Design review of the part built by this model. Coordinates are the model's own, in mm. Face numbers are marked on the shaded views. A direction names the side the tool comes from. Give positions to 0.01 mm unless a question says otherwise; leave off trailing zeros. Loops run counter-clockwise (first coordinate to the right, second up) from the corner with the lowest first, then second, coordinate; pieces in that order, holes last. Notation, with made-up numbers: M -35.5,10.5 L -0.5,10.5 A14 cw -0.5,18.5 Z; hole C 69.5,69.5 d3. An arc over 180 degrees is marked long. Use a Markdown table: item, result. Add a question column.
(1) For probe 1 along X at (y, z) = (11.5, 156.5); probe 2 along Y at (x, z) = (39, -132); probe 3 along Y at (x, z) = (3.5, -138), list the stretches that pass through material, from the lowest coordinate up.
(2) Insertion check: pin 1 Ø1.5 at (x, y) = (26.5, 24.5) entering from -Z; pin 2 Ø1 at (x, y) = (15.5, 28.5) entering from -Z; pin 3 Ø4 at (x, y) = (28.5, -8) entering from +Z. Each pin has a flat end and moves straight along its axis. Give the tip position at first contact, or say it passes through.
(3) For the marked faces 4 and 5, list the 3-axis set-ups (+Z, -Z, +X, -X, +Y, -Y) from which the entire face can be reached by the end or side of a thin tool; tool diameter is ignored.
(4) Add section C-C, the plane y = 27.5. Give the boundary of the cut face in (x, z), then the cut area to 3 significant figures.
(5) Draft analysis for pull direction X (two halves, no side actions). For the marked faces 1, 2 and 3, state which applies: pulls with the +X half, pulls with the -X half, needs draft (parallel to the pull), parting line crosses it, or undercut.
(6) Add section B-B, the plane x = 45.5. Give the boundary of the cut face in (y, z).
(7) Add section D-D, the plane x = 16. Give the boundary of the cut face in (y, z), then the cut area to 3 significant figures.
(8) Add section A-A, the plane z = 120.5. Give the boundary of the cut face in (x, y), then the cut area to 3 significant figures.
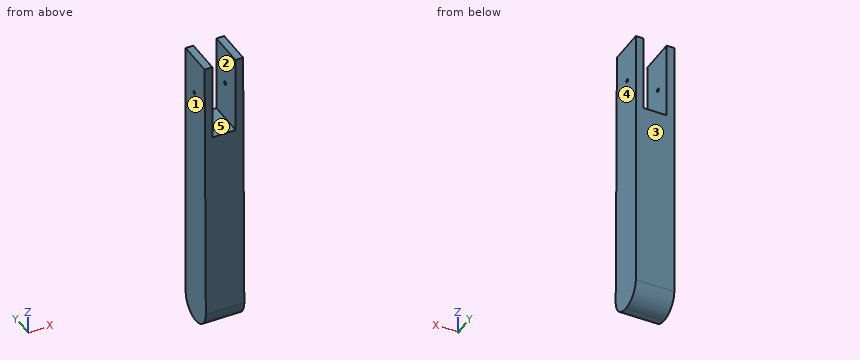
```python
from build123d import *

# Parameters (mm, degrees)
BOSS_EXTRUDE1_DEPTH = 50
SKETCH6_W           = 30
SKETCH6_H           = 100
CUT_EXTRUDE3_DEPTH  = 222.479310794
SKETCH5_R           = 2.25
CUT_EXTRUDE2_DEPTH  = 219.649468957


with BuildPart() as part:
    # Sketch1 → Boss-Extrude1 (new body)
    with BuildSketch(Plane(origin=(0, 0, 0), x_dir=(0, 0, -1), z_dir=(1, 0, 0))):
        with BuildLine():
            Line((140.111731844, 35.418994413), (-209.888268156, 35.418994413))
            Line((-209.888268156, 35.418994413), (-209.888268156, 13.43575419))
            Line((-209.888268156, 13.43575419), (-209.888268156, -11.56424581))
            Line((-209.888268156, -11.56424581), (139.680798176, -14.577291234))
            ThreePointArc((139.680798176, -14.577291234), (115.112660449, 10.634469251), (140.111731844, 35.418994413))
        make_face()
        with BuildLine():
            Line((140.111731844, -14.581005587), (140.111731844, 35.418994413))
            ThreePointArc((140.111731844, 35.418994413), (115.112660449, 10.634469251), (139.680798176, -14.577291234))
            Line((139.680798176, -14.577291234), (140.111731844, -14.581005587))
        make_face()
        with BuildLine():
            ThreePointArc((165.111731844, 10.418994413), (157.789401373, 28.096663943), (140.111731844, 35.418994413))
            Line((140.111731844, 35.418994413), (140.111731844, -14.581005587))
            ThreePointArc((140.111731844, -14.581005587), (157.789401373, -7.258675116), (165.111731844, 10.418994413))
        make_face()
    extrude(amount=BOSS_EXTRUDE1_DEPTH)

    # Sketch6 → Cut-Extrude3 (cut, through all)
    with BuildSketch(Plane(origin=(0, 35.418994413, 0), x_dir=(1, 0, 0), z_dir=(0, 1, 0))):
        with Locations((25, -159.888268156)):
            Rectangle(SKETCH6_W, SKETCH6_H)
    extrude(amount=-CUT_EXTRUDE3_DEPTH, mode=Mode.SUBTRACT)

    # Sketch5 → Cut-Extrude2 (cut, through all)
    with BuildSketch(Plane(origin=(50, 0, 0), x_dir=(0, 0, -1), z_dir=(1, 0, 0))):
        with Locations((-159.888268156, 13.945126907)):
            Circle(SKETCH5_R)
    extrude(amount=-CUT_EXTRUDE2_DEPTH, mode=Mode.SUBTRACT)


solid = part.part
```
Established:
| question | item | result |
|---|---|---|
| 1 | probe 1 | 0 to 10, 40 to 50 |
| 1 | probe 2 | -14.51 to 35.42 |
| 1 | probe 3 | -14.56 to 35.42 |
| 2 | pin 1 | z = -161.26 |
| 2 | pin 2 | z = -157.89 |
| 2 | pin 3 | z = 109.89 |
| 3 | face 4 | +Z, -Z, +X, +Y, -Y |
| 3 | face 5 | +Z, +Y, -Y |
| 4 | outline | M 0,-158.37 L 50,-158.37 L 50,209.89 L 40,209.89 L 40,109.89 L 10,109.89 L 10,209.89 L 0,209.89 Z |
| 4 | area | 15,400 mm^2 |
| 5 | face 1 | pulls with the -X half |
| 5 | face 2 | undercut |
| 5 | face 3 | needs draft |
| 6 | outline | M -14.58,-140.11 A25 ccw 35.42,-140.11 L 35.42,209.89 L -11.56,209.89 Z; hole C 13.95,159.89 d4.5 |
| 7 | outline | M -14.58,-140.11 A25 ccw 35.42,-140.11 L 35.42,109.89 L -12.43,109.89 Z |
| 7 | area | 13,200 mm^2 |
| 8 | outline | M 0,-12.33 L 10,-12.33 L 10,35.42 L 0,35.42 Z; M 40,-12.33 L 50,-12.33 L 50,35.42 L 40,35.42 Z |
| 8 | area | 955 mm^2 |
